```python
from build123d import *

# Parameters (mm, degrees)
SKETCH1_W           = 30.5
SKETCH1_H           = 8.5
BOSS_EXTRUDE1_DEPTH = 20
SHELL1_T            = -2.5
SKETCH2_W           = 12
SKETCH2_H           = 16
CUT_EXTRUDE2_DEPTH  = 3
SKETCH3_W           = 12
SKETCH3_H           = 4
CUT_EXTRUDE3_DEPTH  = 4
SKETCH4_R           = 1.6
CUT_EXTRUDE4_DEPTH  = 10
FILLET1_R           = 3
FILLET2_R           = 3
FILLET3_R           = 3
FILLET4_R           = 3
SKETCH5_R           = 1.45
CUT_EXTRUDE5_DEPTH  = 29
SKETCH12_W          = 25.5
SKETCH12_H          = 3.5
BOSS_EXTRUDE3_DEPTH = 0.75
SKETCH13_R          = 1.462025065
SKETCH13_R_2        = 1.459070956
CUT_EXTRUDE6_DEPTH  = 2
CUT_EXTRUDE7_START  = -2
CUT_EXTRUDE7_DEPTH  = 5
FILLET5_R           = 1.5
FILLET6_R           = 1.5
FILLET7_R           = 1.5
FILLET8_R           = 1.5
FILLET9_R           = 1
FILLET10_R          = 1
CUT_EXTRUDE8_REACH  = 27.507
SKETCH15_W          = 30.5
SKETCH15_H          = 4.25
FILLET13_R          = 1
FILLET14_R          = 1
FILLET15_R          = 1
CUT_EXTRUDE9_DEPTH  = 1.75


with BuildPart() as part:
    # Sketch1 → Boss-Extrude1 (new body)
    with BuildSketch(Plane.XY):
        Rectangle(SKETCH1_W, SKETCH1_H)
    extrude(amount=BOSS_EXTRUDE1_DEPTH)

    # Shell1
    shell1_openings = [part.faces().sort_by_distance(p)[0] for p in [
        (0, 0, 20),
    ]]
    offset(amount=SHELL1_T, openings=shell1_openings, kind=Kind.INTERSECTION)

    # Sketch2 → Cut-Extrude2 (cut)
    with BuildSketch(Plane.XZ.offset(4.25)):
        with Locations((0, 12)):
            Rectangle(SKETCH2_W, SKETCH2_H)
    extrude(amount=-CUT_EXTRUDE2_DEPTH, mode=Mode.SUBTRACT)

    # Sketch3 → Cut-Extrude3 (cut)
    with BuildSketch(Plane(origin=(0, 4.25, 0), x_dir=(1, 0, 0), z_dir=(0, 1, 0))):
        with Locations((0, -5.25)):
            Rectangle(SKETCH3_W, SKETCH3_H)
    extrude(amount=-CUT_EXTRUDE3_DEPTH, mode=Mode.SUBTRACT)

    # Sketch4 → Cut-Extrude4 (cut)
    with BuildSketch(Plane(origin=(0, 4.25, 0), x_dir=(1, 0, 0), z_dir=(0, 1, 0))):
        with Locations(Location((8.9747, -11.35, 0), (0, 0, 270))):
            Circle(SKETCH4_R)
        with Locations(Location((-9.0253, -11.35, 0), (0, 0, 270))):
            Circle(SKETCH4_R)
    extrude(amount=-CUT_EXTRUDE4_DEPTH, mode=Mode.SUBTRACT)

    # Fillet1
    fillet1_edges = [part.edges().sort_by_distance(p)[0] for p in [
        (15.25, 4.25, 10),
    ]]
    fillet(fillet1_edges, radius=FILLET1_R)

    # Fillet2
    fillet2_edges = [part.edges().sort_by_distance(p)[0] for p in [
        (-15.25, 4.25, 10),
    ]]
    fillet(fillet2_edges, radius=FILLET2_R)

    # Fillet3
    fillet3_edges = [part.edges().sort_by_distance(p)[0] for p in [
        (15.25, -4.25, 10),
    ]]
    fillet(fillet3_edges, radius=FILLET3_R)

    # Fillet4
    fillet4_edges = [part.edges().sort_by_distance(p)[0] for p in [
        (-15.25, -4.25, 10),
    ]]
    fillet(fillet4_edges, radius=FILLET4_R)

    # Sketch5 → Cut-Extrude5 (cut)
    with BuildSketch(Plane(origin=(0, 0, 0), x_dir=(-1, 0, 0), z_dir=(0, 0, -1))):
        with Locations((-10.75, -0.182916649)):
            Circle(SKETCH5_R)
        with Locations((10.75, -0.182916649)):
            Circle(SKETCH5_R)
    extrude(amount=-CUT_EXTRUDE5_DEPTH, mode=Mode.SUBTRACT)

    # Sketch12 → Boss-Extrude3 (add)
    with BuildSketch(Plane.XY.offset(2.5)):
        Rectangle(SKETCH12_W, SKETCH12_H)
    extrude(amount=BOSS_EXTRUDE3_DEPTH)

    # Sketch13 → Cut-Extrude6 (cut)
    with BuildSketch(Plane.XY.offset(4)):
        with Locations((-10.75, -0.182916649)):
            Circle(SKETCH13_R)
        with Locations((10.75, -0.182916649)):
            Circle(SKETCH13_R_2)
    extrude(amount=-CUT_EXTRUDE6_DEPTH, mode=Mode.SUBTRACT)

    # Sketch14 → Cut-Extrude7 (cut)
    with BuildSketch(Plane.XY.offset(4).offset(CUT_EXTRUDE7_START)):
        Polygon((-7.25, -0.182916649), (-9, 2.848172265), (-12.5, 2.848172265), (-14.25, -0.182916649), (-12.5, -3.214005562), (-9, -3.214005562), align=None)
        Polygon((14.25, -0.182916649), (12.5, 2.848172265), (9, 2.848172265), (7.25, -0.182916649), (9, -3.214005562), (12.5, -3.214005562), align=None)
    extrude(amount=CUT_EXTRUDE7_DEPTH, mode=Mode.SUBTRACT)

    # Fillet5
    fillet5_edges = [part.edges().sort_by_distance(p)[0] for p in [
        (6, 3, 7.25),
    ]]
    fillet(fillet5_edges, radius=FILLET5_R)

    # Fillet6
    fillet6_edges = [part.edges().sort_by_distance(p)[0] for p in [
        (-6, 3, 7.25),
    ]]
    fillet(fillet6_edges, radius=FILLET6_R)

    # Fillet7
    fillet7_edges = [part.edges().sort_by_distance(p)[0] for p in [
        (-6, 3, 3.25),
    ]]
    fillet(fillet7_edges, radius=FILLET7_R)

    # Fillet8
    fillet8_edges = [part.edges().sort_by_distance(p)[0] for p in [
        (6, 3, 3.25),
    ]]
    fillet(fillet8_edges, radius=FILLET8_R)

    # Fillet9
    fillet9_edges = [part.edges().sort_by_distance(p)[0] for p in [
        (6, -3, 4),
    ]]
    fillet(fillet9_edges, radius=FILLET9_R)

    # Fillet10
    fillet10_edges = [part.edges().sort_by_distance(p)[0] for p in [
        (-6, -3, 4),
    ]]
    fillet(fillet10_edges, radius=FILLET10_R)

    # Cut-Extrude8: up to this face of the body (flat: up to its plane)
    cut_extrude8_end = Plane(part.part.faces().sort_by_distance((0, 0.887010367, 3.25))[0])
    # Sketch15 → Cut-Extrude8 (cut, up to the picked face)
    with BuildSketch(Plane.XY.offset(20), mode=Mode.PRIVATE) as cut_extrude8_sk1:
        with Locations((0, -2.125)):
            Rectangle(SKETCH15_W, SKETCH15_H)
    cut_extrude8_tool1 = split(extrude(cut_extrude8_sk1.sketch, amount=-CUT_EXTRUDE8_REACH, mode=Mode.PRIVATE), bisect_by=cut_extrude8_end, keep=Keep.BOTH, mode=Mode.PRIVATE)
    add(cut_extrude8_tool1.solids().sort_by(Axis((0, -2.125, 20), (0, 0, -1)))[0], mode=Mode.SUBTRACT)

    # Fillet13
    fillet13_edges = [part.edges().sort_by_distance(p)[0] for p in [
        (14.697196512, 0, 3.25),
    ]]
    fillet(fillet13_edges, radius=FILLET13_R)

    # Fillet14
    fillet14_edges = [part.edges().sort_by_distance(p)[0] for p in [
        (-14.697196512, 0, 3.25),
    ]]
    fillet(fillet14_edges, radius=FILLET14_R)

    # Fillet15
    fillet15_edges = [part.edges().sort_by_distance(p)[0] for p in [
        (-6.432984974, 1.75, 3.25),
        (6.432984974, 1.75, 3.25),
    ]]
    fillet(fillet15_edges, radius=FILLET15_R)

    # Sketch16 → Cut-Extrude9 (cut)
    with BuildSketch(Plane.XZ):
        with BuildLine():
            Line((-10.06119106, 15.213538496), (-10.061191059, 7.486461504))
            ThreePointArc((-10.061191059, 7.486461504), (-13.0253, 11.35), (-10.06119106, 15.213538496))
        make_face()
        with BuildLine():
            Line((10.01059106, 15.213538496), (10.010591059, 7.486461504))
            ThreePointArc((10.010591059, 7.486461504), (12.9747, 11.35), (10.01059106, 15.213538496))
        make_face()
    extrude(amount=-CUT_EXTRUDE9_DEPTH, mode=Mode.SUBTRACT)


solid = part.part
```
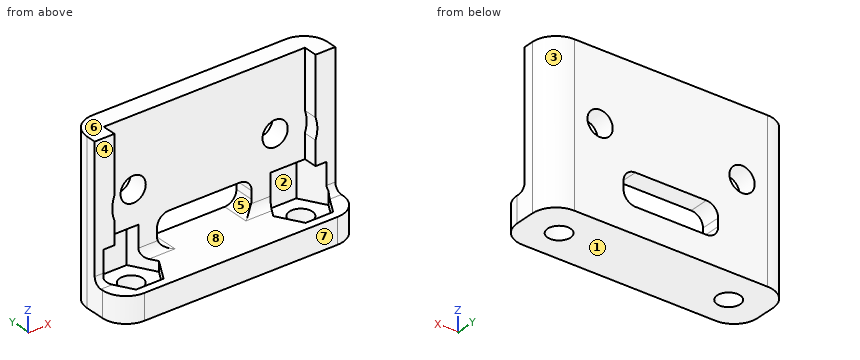
The listing builds one solid part. Answer for the finished solid, in the listing's coordinates (mm). Face numbers are marked on the shaded views. A direction names the side the tool comes from. Give positions to 0.01 mm unless a question says otherwise; leave off trailing zeros. Order: outer loops, then holes, each group sorted by start corner. A loop starts at its lowest first (then second) coordinate and runs counter-clockwise, first axis right, second up. Notation, with made-up numbers: (19.25, -26.5) - (37.25, -26.5) arc R15 ccw to (37.25, -6.5) - close; hole circle Ø7 at (16.25, 37). An arc over 180 degrees is marked (long way). Answer in a Markdown table with one row per item. Add a question column.
Q1. For a pull along Z with two mould halves and no side action, classify the marked faces 6, 7 and 8 as released by +Z, released by -Z, zero draft, split by the parting line, or undercut.
Q2. The part is cut by section A-A (z = 11.35). Determine the outline of the cut face in (x, y).
Q3. Which of the six approach directions +Z, -Z, +X, -X, +Y, -Y give full straight-line access (tool end or side, diameter ignored) to the marked faces 1, 2, 3, 4 and 5?
Q4. Find the intervals of material crossed by line 1 along X through (y, z) = (3.5, 11.25); line 2 along Z through (x, y) = (-2.5, 3); line 3 along Y through (x, z) = (-10.75, 1.15), in increasing order. Write a range as [from, to].
Q5. Given P1, Ø3, axis at x = -9, z = 11.5, coming from the -Y side; P2, Ø0.8, axis at x = 14, z = 10.5, coming from the -Y side; P3, Ø2.5, axis at x = -9.03, z = 11.35, coming from the +Y side; P4, Ø1, axis at x = 11.5, z = 4, coming from the -Y side, each flat-ended and moving along its own axis, determine where each tip first touches the part or whether it passes through.
Q6. The part is cut by section B-B (x = -11.5). Determine the outline of the cut face in (y, z).
Q7. The part is cut by section D-D (x = -6.5). Determine the outline of the cut face in (y, z).
Q8. The part is cut by section C-C (y = 3.5). Determine the outline of the cut face in (x, z), then the cut area to 3 significant figures.
Determined:
| question | item | result |
|---|---|---|
| 1 | face 6 | released by +Z |
| 1 | face 7 | zero draft |
| 1 | face 8 | undercut |
| 2 | outline | (-15.25, 0) - (-13.03, 0) - (-13.03, 1.75) - (-10.63, 1.75) - (-10.63, 4.25) - (-12.25, 4.25) arc R3 ccw to (-15.25, 1.25) - close; (-7.43, 1.75) - (7.37, 1.75) - (7.37, 4.25) - (-7.43, 4.25) - close; (10.57, 1.75) - (12.97, 1.75) - (12.97, 0) - (15.25, 0) - (15.25, 1.25) arc R3 ccw to (12.25, 4.25) - (10.57, 4.25) - close |
| 3 | face 1 | -Z, +X, -X, +Y, -Y |
| 3 | face 2 | none |
| 3 | face 3 | +Z, -Z, +X, +Y |
| 3 | face 4 | +Z, +X, -X, -Y |
| 3 | face 5 | +Y, -Y |
| 4 | line 1 | x = [-14.23, -10.62], [-7.43, 7.38], [10.57, 14.23] |
| 4 | line 2 | z = [0, 3.25], [7.25, 20] |
| 4 | line 3 | y = [-4.25, -1.63], [1.27, 4.25] |
| 5 | P1 | stops at y = 1.75 |
| 5 | P2 | stops at y = 0 |
| 5 | P3 | passes through |
| 5 | P4 | stops at y = 2.85 |
| 6 | outline | (-4.25, 0) - (-1.42, 0) - (-1.42, 2) - (-3.21, 2) - (-3.21, 3.25) - (-4.25, 3.25) - close; (1.06, 0) - (4.25, 0) - (4.25, 20) - (1.75, 20) - (1.75, 7) - (2.85, 7) - (2.85, 2) - (1.06, 2) - close |
| 7 | outline | (-4.25, 0) - (4.25, 0) - (4.25, 20) - (1.75, 20) - (1.75, 4.25) arc R1 cw to (0.75, 3.25) - (-4.25, 3.25) - close |
| 8 | outline | (-14.23, 0) - (14.23, 0) - (14.23, 20) - (-14.23, 20) - close; hole circle Ø3.2 at (-9.03, 11.35); hole (-6, 4.75) arc R1.5 ccw to (-4.5, 3.25) - (4.5, 3.25) arc R1.5 ccw to (6, 4.75) - (6, 5.75) arc R1.5 ccw to (4.5, 7.25) - (-4.5, 7.25) arc R1.5 ccw to (-6, 5.75) - close; hole circle Ø3.2 at (8.97, 11.35) |
| 8 | area | 507 mm² |
